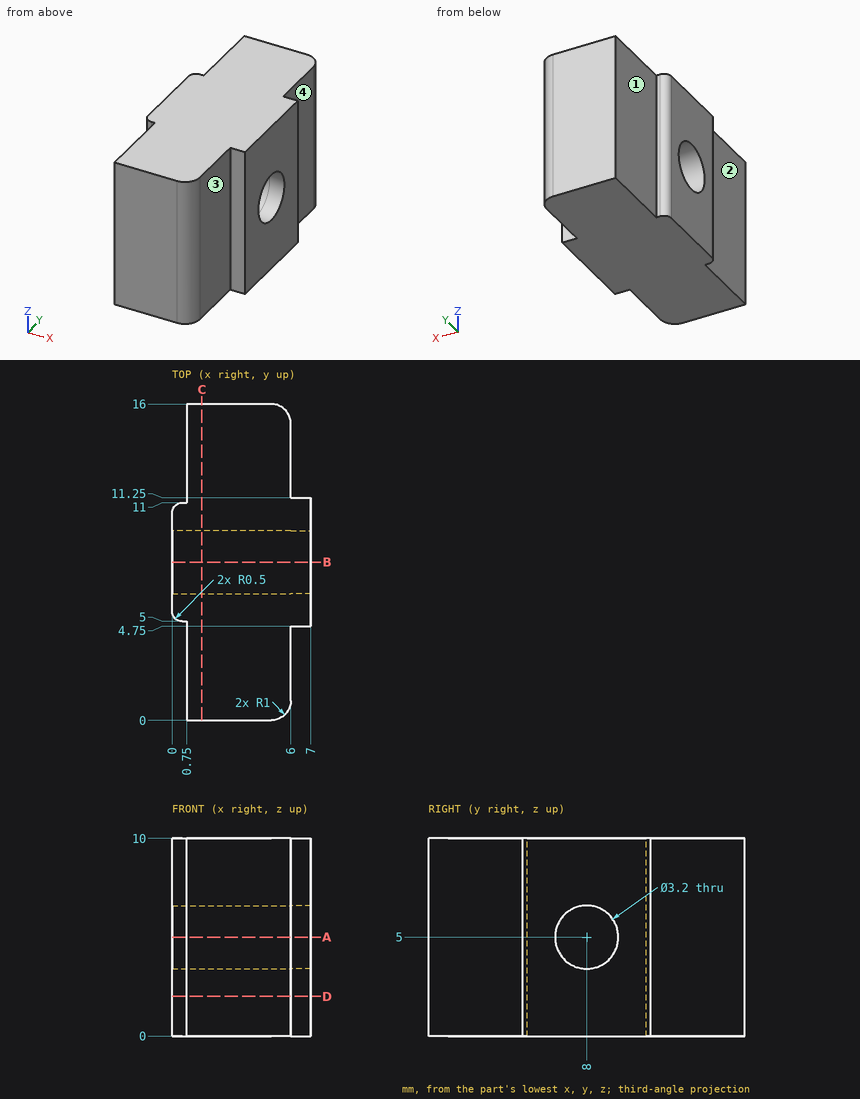
Job drawing, mm, ordinate dimensions from the low corner. One solid piece. A direction names the side the tool comes from. Round coordinates to 2 decimals unless told otherwise and drop trailing zeros. Loops run counter-clockwise (first coordinate to the right, second up) from the corner with the lowest first, then second, coordinate; pieces in that order, holes last. Notation, with made-up numbers: (32, 47) -> (46, 47) arc R20 ccw to (46, 78) -> close; hole circle Ø4 at (43.25, -7). An arc over 180 degrees is marked (long way). Use a Markdown table: item, result.
1) Cut at A-A, the plane z = 5. List the corners of the cut face in (x, y), and give its area (3 significant figures).
The answers:
| item | result |
|---|---|
| outline | (0, 5.5) arc R0.5 ccw to (0.5, 5) -> (0.75, 5) -> (0.75, 0) -> (5, 0) arc R1 ccw to (6, 1) -> (6, 4.75) -> (7, 4.75) -> (7, 6.4) -> (0, 6.4) -> close; (0, 9.6) -> (7, 9.6) -> (7, 11.25) -> (6, 11.25) -> (6, 15) arc R1 ccw to (5, 16) -> (0.75, 16) -> (0.75, 11) -> (0.5, 11) arc R0.5 ccw to (0, 10.5) -> close |
| area | 72.1 mm2 |
2) Drop flat-ended pins along their axis: pin 1 Ø1.5 at (y, z) = (1.5, 6.5) entering from -X; pin 2 Ø4 at (y, z) = (13.5, 3.5) entering from +X; pin 3 Ø0.5 at (x, z) = (6.5, 4) entering from -Y. Give the stop position or say it passes through.
The answers:
| item | result |
|---|---|
| pin 1 | stops at x = 0.75 |
| pin 2 | stops at x = 6 |
| pin 3 | stops at y = 4.75 |
3) Tool access for the marked faces 1, 2, 3 and 4: list every direction of +Z, -Z, +X, -X, +Y, -Y with a clear straight run to the whole face (end or side of a thin tool).
The answers:
| item | result |
|---|---|
| face 1 | +Z, -Z, -X, +Y |
| face 2 | +Z, -Z, -X, -Y |
| face 3 | +Z, -Z, +X, -Y |
| face 4 | +Z, -Z, +X, +Y |
4) Cut at B-B, the plane y = 8. List the corners of the cut face in (x, z).
The answers:
| item | result |
|---|---|
| outline | (0, 0) -> (7, 0) -> (7, 3.4) -> (0, 3.4) -> close; (0, 6.6) -> (7, 6.6) -> (7, 10) -> (0, 10) -> close |
5) Probe line 1 (Z direction, x = 6.75, y = 8); line 2 (X direction, y = 3.75, z = 9.5); line 3 (Y direction, x = 0.5, z = 1). List the from-to ranges inside material, lowest first. Write a range as [from, to].
The answers:
| item | result |
|---|---|
| line 1 | z = [0, 3.4], [6.6, 10] |
| line 2 | x = [0.75, 6] |
| line 3 | y = [5, 11] |
6) Cut at C-C, the plane x = 1.5. List the corners of the cut face in (y, z).
The answers:
| item | result |
|---|---|
| outline | (0, 0) -> (16, 0) -> (16, 10) -> (0, 10) -> close; hole circle Ø3.2 at (8, 5) |
7) Cut at D-D, the plane z = 2. List the corners of the cut face in (x, y), and give its area (3 significant figures).
The answers:
| item | result |
|---|---|
| outline | (0, 5.5) arc R0.5 ccw to (0.5, 5) -> (0.75, 5) -> (0.75, 0) -> (5, 0) arc R1 ccw to (6, 1) -> (6, 4.75) -> (7, 4.75) -> (7, 11.25) -> (6, 11.25) -> (6, 15) arc R1 ccw to (5, 16) -> (0.75, 16) -> (0.75, 11) -> (0.5, 11) arc R0.5 ccw to (0, 10.5) -> close |
| area | 94.5 mm2 |
